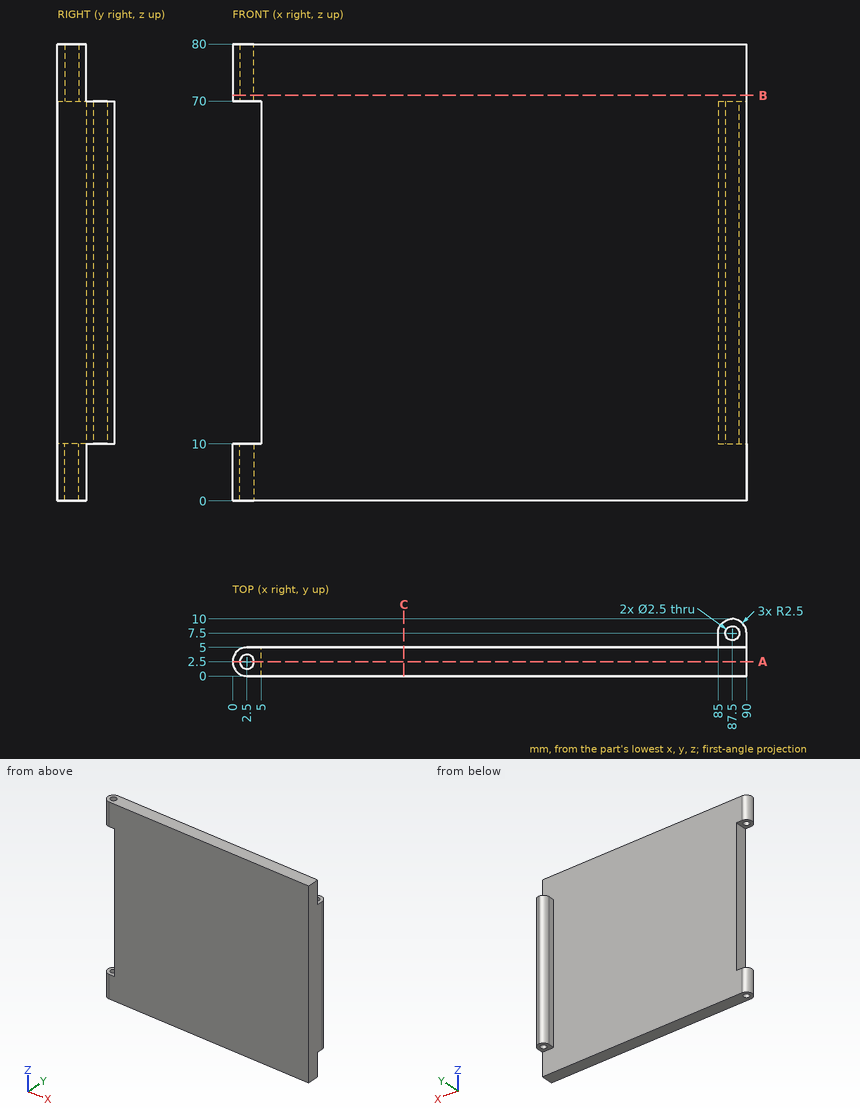
The figure shows three views and two pictorial views of one solid part (mm, origin at its lowest corner). Answer the questions. Round coordinates to 2 decimals unless told otherwise and drop trailing zeros. Order: outer loops, then holes, each group sorted by start corner. A loop starts at its lowest first (then second) coordinate and runs counter-clockwise, first axis right, second up. Notation, with made-up numbers: (45.5, -24) - (77.5, -24) arc R19 ccw to (77.5, -12) - close; hole circle Ø4 at (-23, 29). An arc over 180 degrees is marked (long way). Write item = value, one per line. Start each with the question number.
1) Straight lines are drawn through the part: L1, parallel to X at y = 7.5, z = 50.5; L2, parallel to Y at x = 2.5, z = 2.5; L3, parallel to Y at x = 87.5, z = 57. For each, find the intervals that lie inside material, in ascending order.
2) Section A-A, the plane y = 2.5 is taken. Write down the section's boundary in (x, z), plus the area to 3 significant figures.
3) Section C-C, the plane x = 30 is taken. Write down the section's boundary in (y, z).
4) Given pin 1 (8 mm diameter, centred on x = 59.5, z = 57, fed in from +Y); pin 2 (0.8 mm diameter, centred on y = 6, z = 35, fed in from -X); pin 3 (5.5 mm diameter, centred on y = 1.5, z = 43, fed in from -X), each flat-ended and moving along its own axis, determine where each tip first touches the part or whether it passes through.
5) Section B-B, the plane z = 71 is taken. Write down the section's boundary in (x, y).
Results list:
q1.L1 = 85 to 86.25, 88.75 to 90
q1.L2 = 0 to 1.25, 3.75 to 5
q1.L3 = 0 to 6.25, 8.75 to 10
q2.outline = (0, 0) - (1.25, 0) - (1.25, 10) - (0, 10) - close; (0, 70) - (1.25, 70) - (1.25, 80) - (0, 80) - close; (3.75, 0) - (90, 0) - (90, 80) - (3.75, 80) - (3.75, 70) - (5, 70) - (5, 10) - (3.75, 10) - close
q2.area = 6,850 mm^2
q3.outline = (0, 0) - (5, 0) - (5, 80) - (0, 80) - close
q4.pin_1 = 5
q4.pin_2 = 85
q4.pin_3 = 5
q5.outline = (2.5, 0) - (90, 0) - (90, 5) - (2.5, 5) arc R2.5 ccw to start; hole circle Ø2.5 at (2.5, 2.5)
